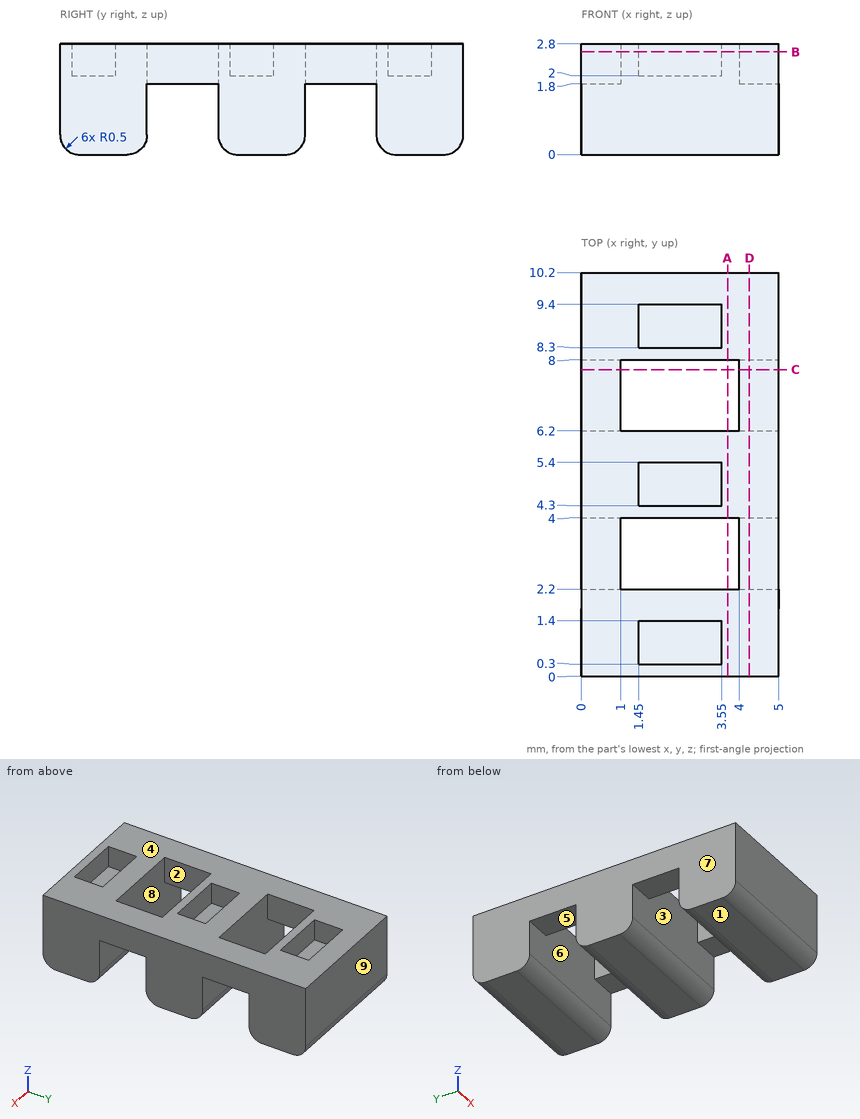
Geometry check sheet. Reference: drawing and pictorial views, mm from the part's lowest x, y, z. A direction names the side the tool comes from. Round coordinates to 2 decimals unless told otherwise and drop trailing zeros. Order: outer loops, then holes, each group sorted by start corner. A loop starts at its lowest first (then second) coordinate and runs counter-clockwise, first axis right, second up. Notation, with made-up numbers: M 44.25,-2 L 70.25,-2 A19 ccw 70.25,28 Z; hole C -8,37.5 d5. An arc over 180 degrees is marked long. Write item = value, one per line.
Q1. Release check for a two-part mould opening along Y. For the marked faces 6, 7, 8 and 9 record: released by +Y, released by -Y, zero draft, split by the parting line, or undercut.
Answer block:
face_6 = undercut
face_7 = zero draft
face_8 = undercut
face_9 = released by +Y
Q2. Section check C-C (y = 7.75). Enter the section's corners in (x, z).
Answer block:
outline = M 0,1.8 L 1,1.8 L 1,2.8 L 0,2.8 Z; M 4,1.8 L 5,1.8 L 5,2.8 L 4,2.8 Z
Q3. Depth check by flat-ended pin: pin 1 Ø0.6 at (x, y) = (2.5, 1) entering from +Z; pin 2 Ø1.1 at (x, y) = (0.5, 3) entering from -Z; pin 3 Ø1.5 at (x, y) = (3, 6.5) entering from -Z. Enter the tip coordinate at first touch or a pass-through.
Answer block:
pin_1 = 2
pin_2 = 1.8
pin_3 = 0
Q4. Section check D-D (x = 4.25). Enter the section's corners in (y, z).
Answer block:
outline = M 0,0.5 A0.5 ccw 0.5,0 L 1.7,0 A0.5 ccw 2.2,0.5 L 2.2,1.8 L 4,1.8 L 4,0.5 A0.5 ccw 4.5,0 L 5.7,0 A0.5 ccw 6.2,0.5 L 6.2,1.8 L 8,1.8 L 8,0.5 A0.5 ccw 8.5,0 L 9.7,0 A0.5 ccw 10.2,0.5 L 10.2,2.8 L 0,2.8 Z
Q5. Section check B-B (z = 2.6). Enter the section's corners in (x, y), plus the area to 3 significant figures.
Answer block:
outline = M 0,0 L 5,0 L 5,10.2 L 0,10.2 Z; hole M 1,2.2 L 4,2.2 L 4,4 L 1,4 Z; hole M 1,6.2 L 4,6.2 L 4,8 L 1,8 Z; hole M 1.45,0.3 L 3.55,0.3 L 3.55,1.4 L 1.45,1.4 Z; hole M 1.45,4.3 L 3.55,4.3 L 3.55,5.4 L 1.45,5.4 Z; hole M 1.45,8.3 L 3.55,8.3 L 3.55,9.4 L 1.45,9.4 Z
area = 33.3 mm^2
Q6. Section check A-A (x = 3.7). Enter the section's corners in (y, z).
Answer block:
outline = M 0,0.5 A0.5 ccw 0.5,0 L 1.7,0 A0.5 ccw 2.2,0.5 L 2.2,2.8 L 0,2.8 Z; M 4,0.5 A0.5 ccw 4.5,0 L 5.7,0 A0.5 ccw 6.2,0.5 L 6.2,2.8 L 4,2.8 Z; M 8,0.5 A0.5 ccw 8.5,0 L 9.7,0 A0.5 ccw 10.2,0.5 L 10.2,2.8 L 8,2.8 Z
Q7. Set-up check for the marked faces 1, 2, 3, 4 and 5: record each of +Z, -Z, +X, -X, +Y, -Y from which the full face is reachable in a straight line by a thin tool's end or side.
Answer block:
face_1 = -Z, +X, -X, +Y, -Y
face_2 = +Z, -Z
face_3 = -Z
face_4 = +Z, +X, -X, +Y, -Y
face_5 = -Z, +X, -X
Q8. Scan lines: line 1 (Y direction, x = 3.5, z = 1.6); line 2 (X direction, y = 8.75, z = 2.4); line 3 (Y direction, x = 1.8, z = 2.35). Record each from-to range of solid material in increasing order.
Answer block:
line_1 = 0 to 2.2, 4 to 6.2, 8 to 10.2
line_2 = 0 to 1.45, 3.55 to 5
line_3 = 0 to 0.3, 1.4 to 2.2, 4 to 4.3, 5.4 to 6.2, 8 to 8.3, 9.4 to 10.2
